Read the model definition and answer for the solid it produces. Units are mm, in the model's axes. Face numbers are marked on the shaded views. Give positions to 0.01 mm unless a question says otherwise; leave off trailing zeros. Loops run counter-clockwise (first coordinate to the right, second up) from the corner with the lowest first, then second, coordinate; pieces in that order, holes last. Notation, with made-up numbers: (-32, -12) - (-16, -12) arc R11 ccw to (-16, 7) - close; hole circle Ø10 at (-28, 27.5). An arc over 180 degrees is marked (long way). Put each result on its own line as item: value. Start each with the question number.
1. Given pin 1 Ø5 at (x, y) = (0, 0.5) entering from -Z; pin 2 Ø3 at (x, z) = (5, 26) entering from -Y, each flat-ended and moving along its own axis, determine where each tip first touches the part or whether it passes through.
2. A cutting plane is placed at B-B, the plane y = -0.75. Determine the outline of the cut face in (x, z).
3. A cutting plane is placed at C-C, the plane z = 26.25. Determine the outline of the cut face in (x, y).
4. A cutting plane is placed at D-D, the plane y = -4. Determine the outline of the cut face in (x, z).
5. For a pull along Y with two mould halves and no side action, classify the marked faces 1, 2 and 3 as released by +Y, released by -Y, zero draft, split by the parting line, or undercut.
6. Consider L1, parallel to X at y = 0, z = 2.25; L2, parallel to Z at x = 6.5, y = 0.25. Determine where each line is inside the solid, lowest interval first. Write a range as from..to.
```python
from build123d import *

# Parameters (mm, degrees)
SKETCH_1_W      = 15
SKETCH_1_H      = 15
SKETCH_1_R      = 5.5
EXTRUDE_1_DEPTH = 30
SKETCH_5_W      = 15
SKETCH_5_H      = 15
EXTRUDE_3_DEPTH = 20
FILLET_2_R      = 7.5


with BuildPart() as part:
    # ｽｹｯﾁ1 → ﾎﾞｽ - 押し出し1 (new body)
    with BuildSketch(Plane.XY):
        Rectangle(SKETCH_1_W, SKETCH_1_H)
        Circle(SKETCH_1_R, mode=Mode.SUBTRACT)
    extrude(amount=EXTRUDE_1_DEPTH)

    # ｽｹｯﾁ5 → ﾎﾞｽ - 押し出し3 (add)
    with BuildSketch(Plane.XY.offset(30)):
        Rectangle(SKETCH_5_W, SKETCH_5_H)
    extrude(amount=-EXTRUDE_3_DEPTH)

    # ﾌｨﾚｯﾄ2
    fillet_2_edges = [part.edges().sort_by_distance(p)[0] for p in [
        (0, -7.5, 30),
        (0, 7.5, 30),
    ]]
    fillet(fillet_2_edges, radius=FILLET_2_R - 0.0001)  # a hair under: the kernel refuses the full size


solid = part.part
```
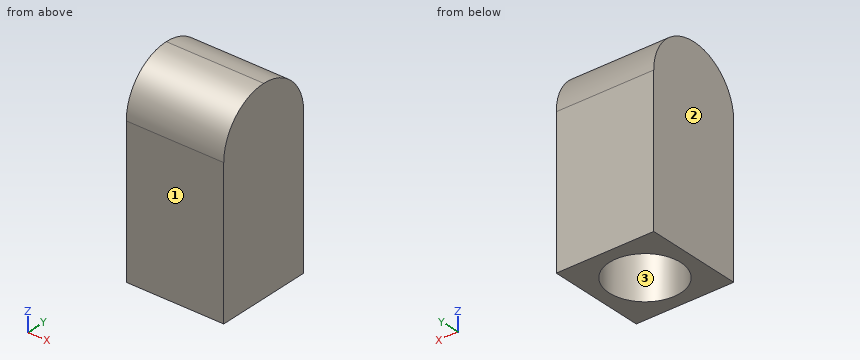
Return value:
1. pin 1: stops at z = 10
1. pin 2: stops at y = -7.23
2. outline: (-7.5, 0) - (-5.45, 0) - (-5.45, 10) - (5.45, 10) - (5.45, 0) - (7.5, 0) - (7.5, 29.96) - (-7.5, 29.96) - close
3. outline: (-7.5, -6.5) - (7.5, -6.5) - (7.5, 6.5) - (-7.5, 6.5) - close
4. outline: (-7.5, 0) - (-3.77, 0) - (-3.77, 10) - (3.77, 10) - (3.77, 0) - (7.5, 0) - (7.5, 28.84) - (-7.5, 28.84) - close
5. face 1: released by -Y
5. face 2: zero draft
5. face 3: undercut
6. L1: x = -7.5..-5.5, 5.5..7.5
6. L2: z = 0..30
